Autodesk Inventor part; units mm, degrees
ref_plane "CP_XY" through (0, 0, 0) normal (1, 0, 0) x (0, 0, -1)
ref_plane "CP_YZ" through (0, 0, 0) normal (0, 0, -1) x (0, 1, 0)
ref_plane "CP_ZX" through (0, 0, 0) normal (0, 1, 0) x (1, 0, 0)
sketch "Sketch_1" plane through (0, 0, 0) normal (0, 0, 1) x (1, 0, 0)
  line L0 (0, 0) -> (-8, 0)
  line L1 (-8, 0) -> (-8, 2.0095)
  line L2 (-8, 2.0095) -> (-7.5095, 2.5)
  line L3 (-7.5095, 2.5) -> (-0.75, 2.5)
  line L4 (-0.75, 2.5) -> (0, 1.75)
  line L5 (0, 1.75) -> (0, 0)
  line L6 (0, 0) -> (-8, 0)
revolve "Revolution1" add sketch "Sketch_1" angle 360 about axis through (0, 0, 0) along (1, 0, 0)
thread "Thread1"
sketch "Sketch_2" plane through (-8, 0, 0) normal (-1, 0, 0) x (0, 1, 0)
  line L0 (-1.25, 0.7217) -> (-1.25, -0.7217)
  line L1 (-1.25, -0.7217) -> (0, -1.4434)
  line L2 (0, -1.4434) -> (1.25, -0.7217)
  line L3 (1.25, -0.7217) -> (1.25, 0.7217)
  line L4 (1.25, 0.7217) -> (0, 1.4434)
  line L5 (0, 1.4434) -> (-1.25, 0.7217)
extrude "Extrusion1" cut sketch "Sketch_2" against normal blind 2
sketch "Sketch_3" plane through (0, 0, 0) normal (0, 0, 1) x (1, 0, 0)
  line L0 (-5.2783, 0) -> (-6, 0)
  line L1 (-6, 0) -> (-6, 1.25)
  line L2 (-6, 1.25) -> (-5.2783, 0)
  line L3 (-5.2783, 0) -> (-6, 0)
revolve "Revolution2" cut sketch "Sketch_3" angle 360 about axis through (-5.2783, 0, 0) along (1, 0, 0)
ref_plane "CP_XY" through (0, 0, 0) normal (1, 0, 0) x (0, 0, -1)
ref_plane "CP_YZ" through (0, 0, 0) normal (0, 0, -1) x (0, 1, 0)
ref_plane "CP_ZX" through (0, 0, 0) normal (0, 1, 0) x (1, 0, 0)
properties part number "SET-SCREW5-8"
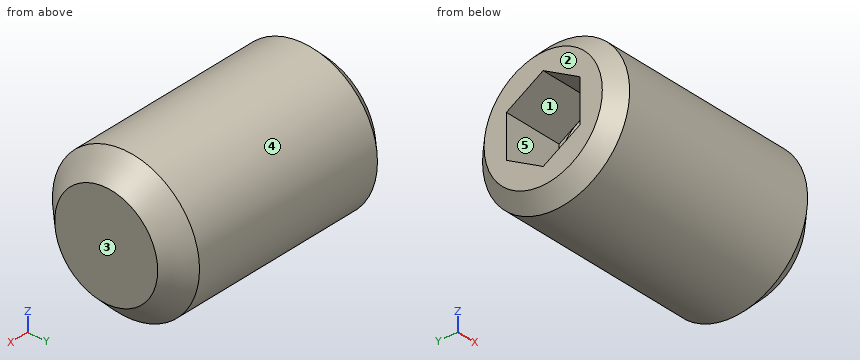
Input: part model. Units: mm. Frame: model coordinates. Face numbers are marked on the shaded views. A direction names the side the tool comes from. Coordinates: 2 decimals unless noted, no trailing zeros. Write each loop counter-clockwise with the first axis right and the second up, starting at its lowest first coordinate (ties: lowest second). Pieces come first, ordered by that corner, then holes.
1) Mould query, pull axis Y, two halves, no side actions, for the marked faces 3, 4 and 5. Classes: pulls with the +Y half, pulls with the -Y half, needs draft (parallel to the pull), parting line crosses it, or undercut.
2) Pin query (flat end, axial travel): pin 1 Ø1.2 at (y, z) = (-0.5, -1) entering from -X; pin 2 Ø0.7 at (y, z) = (0, 0.5) entering from -X. Return the tip coordinate at first contact, or that it passes through.
3) Set-up query: the marked faces 1 and 2. Return all of +Z, -Z, +X, -X, +Y, -Y with unobstructed straight access to the full face (end or side cutting, diameter ignored); none if empty.
4) Section A-A on x = -3.25. Output: boundary loops of the cut face in (y, z).
5) Material intervals for line 1 along Y through (x, z) = (-7, -0.6); line 2 along Y through (x, z) = (-7.25, 0.9); line 3 along Z through (x, y) = (-7, -0.25), sorted ascending.
Check result:
1. face 3: needs draft
1. face 4: parting line crosses it
1. face 5: undercut
2. pin 1: stops at x = -8
2. pin 2: stops at x = -5.77
3. face 1: -X
3. face 2: +Z, -Z, -X, +Y, -Y
4. outline: circle Ø5 at (0, 0)
5. line 1: y = -2.43 to -1.25, 1.25 to 2.43
5. line 2: y = -2.33 to -0.94, 0.94 to 2.33
5. line 3: z = -2.49 to -1.3, 1.3 to 2.49
